Autodesk Inventor part; units mm, degrees
ref_plane "YZ Plane" through (0, 0, 0) normal (1, 0, 0) x (0, 1, 0)
ref_plane "XZ Plane" through (0, 0, 0) normal (0, 1, 0) x (-1, 0, 0)
ref_plane "XY Plane" through (0, 0, 0) normal (0, 0, 1) x (1, 0, 0)
sketch "Sketch1" plane through (0, 0, 0) normal (0, 1, 0) x (-1, 0, 0)
  line L0 (-0.291, 1.3452) -> (-76.291, 1.3452)
  line L1 (-76.291, 1.3452) -> (-76.291, -27.6548)
  line L2 (-76.291, -27.6548) -> (-0.291, -27.6548)
  line L3 (-0.291, -27.6548) -> (-0.291, 1.3452)
  point P0 (0, 0)
  dimension "d0" = 76
  dimension "d1" = 29
extrude "Extrusion1" add sketch "Sketch1" along normal blind 2
sketch "Sketch2" plane through (0, 2, 0) normal (0, 1, 0) x (1, 0, 0)
  line L0 (21.791, 4.6548) -> (46.791, 4.6548)
  line L1 (46.791, 4.6548) -> (46.791, 21.6548)
  line L2 (46.791, 21.6548) -> (21.791, 21.6548)
  line L3 (21.791, 21.6548) -> (21.791, 4.6548)
  line L4 (0.291, 27.6548) -> (0.291, -1.3452)
  line L5 (76.291, -1.3452) -> (76.291, 27.6548)
  line L6 (76.291, 27.6548) -> (0.291, 27.6548)
  point P0 (0, 0)
  point P1 (21.791, 13.1548)
  dimension "d4" = 25
  dimension "d5" = 17
  dimension "d10" = 29.5
  dimension "d18" = 6
extrude "Extrusion2" cut sketch "Sketch2" against normal blind 2
sketch "Sketch3" plane through (0, 2, 0) normal (0, 1, 0) x (1, 0, 0)
  line L0 (48.791, 0.4048) -> (74.291, 0.4048)
  line L1 (74.291, 0.4048) -> (74.291, 25.9048)
  line L2 (74.291, 25.9048) -> (48.791, 25.9048)
  line L3 (48.791, 25.9048) -> (48.791, 0.4048)
  line L4 (76.291, -1.3452) -> (76.291, 27.6548)
  line L5 (46.791, 21.6548) -> (46.791, 4.6548)
  point P0 (0, 0)
  point P1 (74.291, 13.1548)
  point P2 (76.291, 13.1548)
  dimension "d8" = 25.5
  dimension "d27" = 2
extrude "Extrusion3" cut sketch "Sketch3" against normal blind 2
sketch "Sketch4" plane through (0, 0, 0) normal (0, -1, 0) x (1, 0, 0)
  line L0 (74.291, -25.9048) -> (48.791, -25.9048)
  line L1 (48.791, -25.9048) -> (48.791, -0.4048)
  line L2 (48.791, -0.4048) -> (74.291, -0.4048)
  line L3 (74.291, -0.4048) -> (74.291, -25.9048)
  line L4 (46.791, -21.6548) -> (21.791, -21.6548)
  line L5 (21.791, -21.6548) -> (21.791, -4.6548)
  line L6 (21.791, -4.6548) -> (46.791, -4.6548)
  line L7 (46.791, -4.6548) -> (46.791, -21.6548)
  line L8 (76.291, 1.3452) -> (76.291, -27.6548)
  line L9 (0.291, 1.3452) -> (76.291, 1.3452)
  line L10 (0.291, -27.6548) -> (0.291, 1.3452)
  line L11 (76.291, -27.6548) -> (0.291, -27.6548)
  line L12 (21.791, -27.6548) -> (46.791, -27.6548)
  line L13 (46.791, -27.6548) -> (46.791, 1.3452)
  line L14 (46.791, 1.3452) -> (21.791, 1.3452)
  line L15 (21.791, 1.3452) -> (21.791, -27.6548)
  point P0 (0, 0)
  point P1 (46.791, -21.6548)
  point P2 (21.791, 1.3452)
  point P3 (21.791, -4.6548)
  point P4 (46.791, -4.6548)
extrude "Extrusion4" cut sketch "Sketch4" against normal blind 0.5 contours L13 L11 L15 L4 | L6 L15 L9 L13
sketch "Sketch9" plane through (0, 2, 0) normal (0, 1, 0) x (1, 0, 0)
  line L0 (48.791, 25.9048) -> (74.291, 25.9048)
  line L1 (74.291, 25.9048) -> (74.291, 0.4048)
  line L2 (74.291, 0.4048) -> (48.791, 0.4048)
  line L3 (48.791, 0.4048) -> (48.791, 25.9048)
  line L4 (21.791, 21.6548) -> (46.791, 21.6548)
  line L5 (46.791, 21.6548) -> (46.791, 4.6548)
  line L6 (46.791, 4.6548) -> (21.791, 4.6548)
  line L7 (21.791, 4.6548) -> (21.791, 21.6548)
  line L8 (76.291, -1.3452) -> (76.291, 27.6548)
  line L9 (76.291, 27.6548) -> (0.291, 27.6548)
  line L10 (0.291, 27.6548) -> (0.291, -1.3452)
  line L11 (0.291, -1.3452) -> (76.291, -1.3452)
  line L12 (46.791, 15.6362) -> (21.791, 15.6362)
  line L13 (21.791, 21.6548) -> (46.791, 21.6548)
  line L14 (21.791, 4.6548) -> (21.791, 21.6548)
  line L15 (46.791, 21.6548) -> (46.791, 4.6548)
  point P0 (0, 0)
extrude "Extrusion9" add sketch "Sketch9" against normal blind 0.4 contours L4 L5 L12 L7
sketch "Sketch10" plane through (0, 0, 0) normal (0, -1, 0) x (1, 0, 0)
  line L0 (46.791, 1.3452) -> (46.791, -27.6548)
  line L1 (76.291, -27.6548) -> (46.791, -27.6548)
  line L2 (76.291, 1.3452) -> (76.291, -27.6548)
  line L3 (46.791, 1.3452) -> (76.291, 1.3452)
  line L4 (74.291, -25.9048) -> (48.791, -25.9048)
  line L5 (48.791, -25.9048) -> (48.791, -0.4048)
  line L6 (48.791, -0.4048) -> (74.291, -0.4048)
  line L7 (74.291, -0.4048) -> (74.291, -25.9048)
  line L8 (47.791, -26.9048) -> (75.291, -26.9048)
  line L9 (75.291, -26.9048) -> (75.291, 0.5952)
  line L10 (75.291, 0.5952) -> (47.791, 0.5952)
  line L11 (47.791, 0.5952) -> (47.791, -26.9048)
  line L12 (47.791, -26.9048) -> (47.791, -27.6548)
  line L13 (47.791, 0.5952) -> (47.791, 1.3452)
  point P0 (0, 0)
  dimension "d32" = 1
extrude "Extrusion10" add sketch "Sketch10" along normal blind 4 contours L3 L2 L1 L12 L8 L9 L10 L13 | L10 L9 L8 L11
sketch "Sketch13" plane through (0, 0.5, 0) normal (0, -1, 0) x (1, 0, 0)
  circle A0 centre (44.791, -1.6548) radius 1.25
  circle A1 centre (23.791, -1.6548) radius 1.25
  circle A2 centre (44.791, -24.6548) radius 1.25
  circle A3 centre (23.791, -24.6548) radius 1.25
  line L0 (44.791, -1.6548) -> (23.791, -1.6548) construction
  line L1 (46.791, -4.6548) -> (21.791, -4.6548) construction
  point P0 (0, 0)
  point P1 (51.5193, 88.3762)
  point P2 (34.291, -1.6548)
  point P3 (34.291, -4.6548)
  point P4 (21.791, 1.3452)
  dimension "d44" = 2.5
  dimension "d45" = 2.5
  dimension "d46" = 2.5
  dimension "d47" = 2.5
  dimension "d48" = 23
  dimension "d49" = 21
  dimension "d50" = 3
extrude "Extrusion13" add sketch "Sketch13" along normal blind 1
sketch "Sketch14" plane through (0, 1.6, 0) normal (0, -1, 0) x (1, 0, 0)
  line L0 (46.791, -15.6362) -> (46.791, -21.6548)
  line L1 (46.791, -15.6362) -> (21.791, -15.6362)
  line L2 (21.791, -21.6548) -> (21.791, -15.6362)
  line L3 (46.791, -21.6548) -> (21.791, -21.6548)
  line L4 (46.791, -17.6362) -> (21.791, -17.6362)
  point P0 (0, 0)
  dimension "d53" = 2
extrude "Extrusion14" cut sketch "Sketch14" against normal blind 1 contours L0 L4 L2 L1
properties part number "pokrywka2"
CAD build for the part. Positions are in the model's coordinates, mm. A direction names the side the tool comes from. Coordinates: 2 decimals unless noted, no trailing zeros. Order: outer loops, then holes, each group sorted by start corner. A loop starts at its lowest first (then second) coordinate and runs counter-clockwise, first axis right, second up. Notation, with made-up numbers: (65, 9) -> (110, 9) arc R11 cw to (110, 30) -> close; hole circle Ø5 at (13, -38.75). An arc over 180 degrees is marked (long way). Use one line per item in the form item = value. Start each with the question number.
1) Band-saw the part on A-A on z = -16.75. Give the cut face in (x, y).
2) Drill centre lines: L1, parallel to Z at x = 73.5, y = 0.9; L2, parallel to X at y = -1.55, z = -16.75; L3, parallel to X at y = 0.9, z = -6. Where is each one in solid material? Low to high. Write a range as [from, to].
3) Pull direction X, two halves, no side cores. Call faces 1 (the flat face through (75, -4, -13)), 2 (the flat face through (76.291, -1, -13)), 3 (the flat face through (0.291, 1, -13)), 4 (the flat face through (34, 0.5, -25)): +X half, -X half, draft (parallel to the pull), parting line (faces both ways), or undercut.
4) Tool access for faces 5 (the flat face through (24, -0.5, -25)), 6 (the flat face through (74.291, -1, -13)), 7 (the cylindrical face through (22.87, 0.01, -25.5)): list every direction of +Z, -Z, +X, -X, +Y, -Y with a clear straight run to the whole face (end or side of a thin tool).
5) Band-saw the part on D-D on x = 29. Give the cut face in (y, z), then the cut area to 3 significant figures.
6) Drop flat-ended pins along their axis: pin 1 (17 mm diameter, centred on x = 8.5, z = -17, fed in from -Y); pin 2 (1.5 mm diameter, centred on y = -2.5, z = -15.5, fed in from -X); pin 3 (3 mm diameter, centred on x = 40.5, z = 0, fed in from -Y); pin 4 (3 mm diameter, centred on y = -1, z = -8, fed in from -X). Give the stop position or say it passes through.
7) Band-saw the part on C-C on y = -1.4. Give the cut face in (x, z).
8) Band-saw the part on B-B on x = 52. Give the cut face in (y, z).
Entries:
q1.outline = (0.29, 0) -> (21.79, 0) -> (21.79, 2) -> (0.29, 2) -> close; (46.79, 0) -> (47.79, 0) -> (47.79, -4) -> (48.79, -4) -> (48.79, 2) -> (46.79, 2) -> close; (74.29, -4) -> (76.29, -4) -> (76.29, 2) -> (74.29, 2) -> close
q2.L1 = [-27.65, -25.9], [-0.4, 1.35]
q2.L2 = [47.79, 48.79], [74.29, 76.29]
q2.L3 = [0.29, 21.79], [46.79, 48.79], [74.29, 76.29]
q3.face_1 = draft
q3.face_2 = +X half
q3.face_3 = -X half
q3.face_4 = undercut
q4.face_5 = +Z, -Z, -X, -Y
q4.face_6 = +Y, -Y
q4.face_7 = -Y
q5.outline = (0.5, -27.65) -> (2, -27.65) -> (2, -17.64) -> (1.6, -17.64) -> (1.6, -21.65) -> (0.5, -21.65) -> close; (0.5, -4.65) -> (2, -4.65) -> (2, 1.35) -> (0.5, 1.35) -> close
q5.area = 19.6 mm2
q6.pin_1 = 0
q6.pin_2 = 47.79
q6.pin_3 = 0.5
q6.pin_4 = 0.29
q7.outline = (47.79, -27.65) -> (76.29, -27.65) -> (76.29, 1.35) -> (47.79, 1.35) -> close; hole (48.79, -25.9) -> (74.29, -25.9) -> (74.29, -0.4) -> (48.79, -0.4) -> close
q8.outline = (-4, -27.65) -> (2, -27.65) -> (2, -25.9) -> (-4, -25.9) -> close; (-4, -0.4) -> (2, -0.4) -> (2, 1.35) -> (-4, 1.35) -> close
